from build123d import *

# Parameters (mm, degrees)
BOSS_EXTRUDE1_DEPTH = 5
BOSS_EXTRUDE2_DEPTH = 5
BOSS_EXTRUDE4_DEPTH = 5
BOSS_EXTRUDE6_DEPTH = 5
SKETCH9_R           = 2
BOSS_EXTRUDE7_DEPTH = 5


with BuildPart() as part:
    # Sketch1 → Boss-Extrude1 (new body)
    with BuildSketch(Plane.XY):
        with BuildLine():
            Line((-4.859145774, 0.392452951), (-6.826544894, 0.392452951))
            ThreePointArc((-6.826544894, 0.392452951), (-3.265295394, 1.642452951), (-6.826544894, 2.892452951))
            Line((-6.826544894, 2.892452951), (-4.859145774, 2.892452951))
            Line((-4.859145774, 2.892452951), (-3.950967614, 1.642452951))
            Line((-3.950967614, 1.642452951), (-4.859145774, 0.392452951))
        make_face()
    extrude(amount=BOSS_EXTRUDE1_DEPTH)

    # Sketch2 → Boss-Extrude2 (add)
    with BuildSketch(Plane(origin=(0, 0, 0), x_dir=(-1, 0, 0), z_dir=(0, 0, -1))):
        with BuildLine():
            ThreePointArc((3.704045895, 0.392452951), (3.265295394, 1.642452951), (3.704045895, 2.892452951))
            Line((3.704045895, 2.892452951), (-1.927293689, 2.892452951))
            Line((-1.927293689, 2.892452951), (-1.927293689, 0.392452951))
            Line((-1.927293689, 0.392452951), (3.704045895, 0.392452951))
        make_face()
    extrude(amount=-BOSS_EXTRUDE2_DEPTH)

    # Sketch7 → Boss-Extrude4 (add)
    with BuildSketch(Plane(origin=(0, 0, 0), x_dir=(-1, 0, 0), z_dir=(0, 0, -1))):
        with BuildLine():
            ThreePointArc((-1.927293689, 2.892452951), (-4.011161168, 1.936887773), (-4.646831412, -0.265731537))
            ThreePointArc((-4.646831412, -0.265731537), (-4.049138928, -1.606910585), (-2.846528345, -2.449362561))
            ThreePointArc((-2.846528345, -2.449362561), (-2.393666578, -2.567712418), (-1.927293689, -2.607547049))
            Line((-1.927293689, -2.607547049), (-1.927293689, -0.107547049))
            add(Edge.make_bspline(
                [(-1.927293689, 0.392452951), (-2.027068627, 0.287688693), (-2.096009728, 0.076120474), (-1.927293689, -0.107547049)],
                knots=[0, 0, 0, 0, 1, 1, 1, 1], degree=3))
            Line((-1.927293689, 0.392452951), (-1.927293689, 2.892452951))
        make_face()
        with BuildLine():
            Line((-1.927293689, -0.107547049), (-1.927293689, -2.607547049))
            ThreePointArc((-1.927293689, -2.607547049), (-0.073244067, -1.88855665), (0.811319098, -0.107547049))
            Line((0.811319098, -0.107547049), (-1.927293689, -0.107547049))
        make_face()
        with BuildLine():
            Line((-5.566066067, -5.607547049), (1.516820501, -5.607547049))
            ThreePointArc((1.516820501, -5.607547049), (2.192724029, -5.344537158), (2.51308893, -4.69385589))
            Line((2.51308893, -4.69385589), (2.816301333, -1.19385589))
            ThreePointArc((2.816301333, -1.19385589), (2.557023013, -0.431643521), (1.820032904, -0.107547049))
            Line((1.820032904, -0.107547049), (0.811319098, -0.107547049))
            ThreePointArc((0.811319098, -0.107547049), (-0.073244067, -1.88855665), (-1.927293689, -2.607547049))
            Line((-1.927293689, -2.607547049), (0.210410566, -2.607547049))
            ThreePointArc((0.210410566, -2.607547049), (0.351831922, -2.666125693), (0.410410566, -2.807547049))
            Line((0.410410566, -2.807547049), (0.410410566, -2.907547049))
            ThreePointArc((0.410410566, -2.907547049), (0.351831922, -3.048968405), (0.210410566, -3.107547049))
            Line((0.210410566, -3.107547049), (-2.82745328, -3.107547049))
            Line((-2.82745328, -3.107547049), (-5.566066067, -3.107547049))
            Line((-5.566066067, -3.107547049), (-5.566066067, -5.607547049))
        make_face()
    extrude(amount=-BOSS_EXTRUDE4_DEPTH)

    # Sketch8 → Boss-Extrude6 (add)
    with BuildSketch(Plane(origin=(0, 0, 0), x_dir=(-1, 0, 0), z_dir=(0, 0, -1))):
        with BuildLine():
            Line((-10.013976401, -2.607547049), (-5.825134583, -2.607547049))
            ThreePointArc((-5.825134583, -2.607547049), (-3.075134583, 0.142452951), (-5.825134583, 2.892452951))
            Line((-5.825134583, 2.892452951), (-16.568194085, 2.892452951))
            ThreePointArc((-16.568194085, 2.892452951), (-19.02871008, 0.014266669), (-16.282434429, -2.592659737))
            add(Edge.make_bspline(
                [(-16.515824565, -3.107547049), (-16.307464717, -3.001414127), (-16.25870467, -2.690751367), (-16.282434429, -2.592659737)],
                knots=[0, 0, 0, 0, 1, 1, 1, 1], degree=3))
            Line((-16.515824565, -3.107547049), (-19.631835761, -3.107547049))
            Line((-19.631835761, -3.107547049), (-19.631835761, -5.607101349))
            Line((-19.631835761, -5.607101349), (-16.213002559, -5.607101349))
            Line((-16.213002559, -5.607101349), (-15.606969091, -5.607101349))
            ThreePointArc((-15.606969091, -5.607101349), (-15.351610534, -5.536975757), (-15.167880656, -5.346269377))
            Line((-15.167880656, -5.346269377), (-14.894043788, -4.843532439))
            ThreePointArc((-14.894043788, -4.843532439), (-14.343989393, -5.402533166), (-13.587014521, -5.607547049))
            Line((-13.587014521, -5.607547049), (-12.513976401, -5.607547049))
            Line((-12.513976401, -5.607547049), (-10.013976401, -5.607547049))
            Line((-10.013976401, -5.607547049), (-5.566066067, -5.607547049))
            Line((-5.566066067, -5.607547049), (-5.566066067, -3.107547049))
            Line((-5.566066067, -3.107547049), (-10.013976401, -3.107547049))
            add(Edge.make_bspline(
                [(-10.013976401, -3.107547049), (-10.219087549, -2.993746895), (-10.173628104, -2.655391711), (-10.013976401, -2.607547049)],
                knots=[0, 0, 0, 0, 1, 1, 1, 1], degree=3))
        make_face()
        with BuildLine():
            ThreePointArc((-10.013976401, -0.092659737), (-12.028194826, -0.96690939), (-12.765194219, -3.035295286))
            add(Edge.make_bspline(
                [(-12.765194219, -3.035295286), (-12.975821702, -1.859806275), (-13.402295233, -1.005750906), (-13.973446446, -0.404146587)],
                knots=[0.010692284, 0.010692284, 0.010692284, 0.010692284, 0.535473495, 0.535473495, 0.535473495, 0.535473495], degree=3))
            ThreePointArc((-13.973446446, -0.404146587), (-14.304026887, -0.17382538), (-14.698670302, -0.092659737))
            Line((-14.698670302, -0.092659737), (-16.282434429, -0.092659737))
            add(Edge.make_bspline(
                [(-16.282434429, 0.407340263), (-16.503590414, 0.314326842), (-16.500815382, 0.048327648), (-16.282434429, -0.092659737)],
                knots=[0, 0, 0, 0, 1, 1, 1, 1], degree=3))
            Line((-16.282434429, 0.407340263), (-8.563747371, 0.407340263))
            Line((-8.563747371, 0.407340263), (-5.825134583, 0.407340263))
            add(Edge.make_bspline(
                [(-5.825134583, 0.407340263), (-5.661105782, 0.377805029), (-5.562243404, 0.004958528), (-5.825134583, -0.092659737)],
                knots=[0, 0, 0, 0, 1, 1, 1, 1], degree=3))
            Line((-5.825134583, -0.092659737), (-10.013976401, -0.092659737))
        make_face(mode=Mode.SUBTRACT)
    extrude(amount=-BOSS_EXTRUDE6_DEPTH)

    # Sketch9 → Boss-Extrude7 (add)
    # profile 1 of 2: a face of its own
    with BuildSketch(Plane(origin=(0, 0, 0), x_dir=(-1, 0, 0), z_dir=(0, 0, -1))):
        with BuildLine():
            ThreePointArc((4.246387568, -5.256955873), (4.08434285, -3.906172489), (4.823858789, -2.764248492))
            Line((4.823858789, -2.764248492), (4.472208625, -2.764248492))
            ThreePointArc((4.472208625, -2.764248492), (3.970628521, -2.629359698), (3.604363487, -2.26108329))
            Line((3.604363487, -2.26108329), (2.776044941, -0.814219613))
            ThreePointArc((2.776044941, -0.814219613), (2.814457703, -1.002098868), (2.816301333, -1.19385589))
            Line((2.816301333, -1.19385589), (2.515486097, -4.66618525))
            ThreePointArc((2.515486097, -4.66618525), (3.341666009, -5.076630322), (4.246387568, -5.256955873))
        make_face()
    # profile 2 of 2: a face of its own
    with BuildSketch(Plane(origin=(0, 0, 0), x_dir=(-1, 0, 0), z_dir=(0, 0, -1))):
        with Locations((6.032742451, -4.357547049)):
            Circle(SKETCH9_R)
        Polygon((6.805727945, -3.407931817), (5.596844283, -3.213314358), (4.823858789, -4.16292959), (5.259756957, -5.307162281), (6.468640619, -5.501779739), (7.241626113, -4.552164507), align=None, mode=Mode.SUBTRACT)
    extrude(amount=-BOSS_EXTRUDE7_DEPTH)


solid = part.part
For this review, take the finished solid that the model builds, in its own axes (mm). A direction names the side the tool comes from. Coordinates: 2 decimals unless noted, no trailing zeros. Write each loop counter-clockwise with the first axis right and the second up, starting at its lowest first coordinate (ties: lowest second). Pieces come first, ordered by that corner, then holes. Notation, with made-up numbers: (24.5, 76.25) -> (71.5, 76.25) arc R25 cw to (71.5, 103.25) -> close; hole circle Ø6 at (7, 59.5). An arc over 180 degrees is marked (long way). Write each question's results on one line, items separated by ' | '. Start each with the question number.
1) Consider section B-B (x = 17). Write out the cut boundary in (y, z).
2) Consider section C-C (y = 2.5). Write out the cut boundary in (x, z).
3) Consider section A-A (x = 9.75). Write out the cut boundary in (y, z).
4) Insertion check: pin 1 (0.9 mm diameter, centred on x = 19, z = 2, fed in from +Y); pin 2 (1.5 mm diameter, centred on x = 12, z = 2.5, fed in from -Y); pin 3 (2.5 mm diameter, centred on x = 8.5, z = 3.5, fed in from +Y). Each pin has a flat end and moves straight along its axis. Give the tip position at first contact, or say it passes through.
5) For faces 1 (the face through (-6.85, -5.034, 2.465)), 2 (the face through (6, -5.608, 2)), 3 (the face through (4.756, 2.676, 2.465)), 4 (the face through (-4.411, 2.276, 2.465)), list the 3-axis set-ups (+Z, -Z, +X, -X, +Y, -Y) from which the entire face can be reached by the end or side of a thin tool; tool diameter is ignored.
6) Consider section D-D (z = 1). Give the number of separate pieces and of enclosed holes in the cut face, plus the area to 3 significant figures.
7) The part is to be moulded in two halves that separate along Y. For faces 5 (the face through (18, -3.108, 2)), 6 (the face through (19.632, -4, 2)), 7 (the face through (-2.185, -5.352, 2.465)), 8 (the face through (2.969, 2.688, 2.465)), say which applies: +Y half, -Y half, draft (parallel to the pull), parting line (faces both ways), or undercut.
8) Wall thickness on L1, parallel to Y at x = 7.25, z = 3.1; L2, parallel to X at y = 0.25, z = 4.7; L3, parallel to X at y = 0, z = 2.2: over which ranges is each line inside the solid? List them lowest first. Write a range as [from, to].
Geometry says:
1) outline: (-5.61, 0) -> (-3.11, 0) -> (-3.11, 5) -> (-5.61, 5) -> close; (-2.5, 0) -> (2.81, 0) -> (2.81, 5) -> (-2.5, 5) -> close
2) outline: (-4.57, 0) -> (3.34, 0) -> (3.34, 5) -> (-4.57, 5) -> close; (4.41, 0) -> (17.72, 0) -> (17.72, 5) -> (4.41, 5) -> close
3) outline: (-5.61, 0) -> (-3.11, 0) -> (-3.11, 5) -> (-5.61, 5) -> close; (-2.61, 0) -> (-0.09, 0) -> (-0.09, 5) -> (-2.61, 5) -> close; (0.41, 0) -> (2.89, 0) -> (2.89, 5) -> (0.41, 5) -> close
4) pin 1: y = 1.71 | pin 2: y = -5.61 | pin 3: y = 2.89
5) face 1: +Z, -Z | face 2: +Z, -Z, +X, -Y | face 3: +Z, -Z, +Y | face 4: +Z, -Z, -X
6) separate pieces: 1 | enclosed holes: 3 | area: 184 mm^2
7) face 5: undercut | face 6: draft | face 7: -Y half | face 8: +Y half
8) L1: [-5.61, -3.11], [-2.61, -0.09], [0.41, 2.89] | L2: [-6.7, -3.83], [2.01, 5.68], [16.44, 19.03] | L3: [-6.41, -4.12], [2, 5.7], [16.38, 19.03]
